```python
from build123d import *

# Parameters (mm, degrees)
SKETCH_1_W          = 20
SKETCH_1_H          = 10
EXTRUDE_1_DEPTH     = 3
SKETCH_2_W          = 20
SKETCH_2_H          = 3
EXTRUDE_2_DEPTH     = 18
SKETCH_3_W          = 16
SKETCH_3_H          = 12
CUT_EXTRUDE_1_DEPTH = 8
EXTRUDE_3_DEPTH     = 3
SKETCH_5_R          = 1.05
CUT_EXTRUDE_2_DEPTH = 10
FILLET_2_R          = 1
FILLET_3_R          = 1
FILLET_4_R          = 1
SKETCH_6_W          = 20
SKETCH_6_H          = 21
CUT_EXTRUDE_3_DEPTH = 10
SKETCH_7_W          = 24
SKETCH_7_H          = 24
EXTRUDE_4_DEPTH     = 3
SKETCH_8_W          = 24
SKETCH_8_H          = 3
EXTRUDE_5_DEPTH     = 7
SKETCH_9_W          = 20
SKETCH_9_H          = 18
CUT_EXTRUDE_4_DEPTH = 7
SKETCH_10_W         = 32
SKETCH_10_H         = 7
EXTRUDE_6_DEPTH     = 3
SKETCH_11_R         = 1.1
CUT_EXTRUDE_5_DEPTH = 4


with BuildPart() as part:
    # 草图1 → 凸台-拉伸1 (new body)
    with BuildSketch(Plane.XY):
        with Locations((10, 5)):
            Rectangle(SKETCH_1_W, SKETCH_1_H)
    extrude(amount=EXTRUDE_1_DEPTH)

    # 草图2 → 凸台-拉伸2 (add)
    with BuildSketch(Plane.XY.offset(3)):
        with Locations((10, 8.5)):
            Rectangle(SKETCH_2_W, SKETCH_2_H)
    extrude(amount=EXTRUDE_2_DEPTH)

    # 草图3 → 切除-拉伸1 (cut)
    with BuildSketch(Plane.XZ.offset(-7)):
        with Locations((10, 12)):
            Rectangle(SKETCH_3_W, SKETCH_3_H)
    extrude(amount=-CUT_EXTRUDE_1_DEPTH, mode=Mode.SUBTRACT)

    # 草图4 → 凸台-拉伸3 (add)
    with BuildSketch(Plane.XZ.offset(-7)):
        Polygon((0, 21), (-3.5, 21), (-3.5, 38), (23.5, 38), (23.5, 21), align=None)
    extrude(amount=-EXTRUDE_3_DEPTH)

    # 草图5 → 切除-拉伸2 (cut)
    with BuildSketch(Plane.XZ.offset(-7)):
        with Locations((-0.5, 23.5)):
            Circle(SKETCH_5_R)
        with Locations((20.5, 23.5)):
            Circle(SKETCH_5_R)
        with Locations((20.5, 35.5)):
            Circle(SKETCH_5_R)
        with Locations((-0.5, 35.5)):
            Circle(SKETCH_5_R)
    extrude(amount=-CUT_EXTRUDE_2_DEPTH, mode=Mode.SUBTRACT)

    # 圆角2
    fillet_2_edges = [part.edges().sort_by_distance(p)[0] for p in [
        (10, 0, 3),
    ]]
    fillet(fillet_2_edges, radius=FILLET_2_R)

    # 圆角3
    fillet_3_edges = [part.edges().sort_by_distance(p)[0] for p in [
        (0, 4, 3),
        (20, 4, 3),
        (20, 0, 1),
        (20, 0.292893219, 2.707106781),
        (0, 0, 1),
        (0, 0.292893219, 2.707106781),
    ]]
    fillet(fillet_3_edges, radius=FILLET_3_R)

    # 圆角4
    fillet_4_edges = [part.edges().sort_by_distance(p)[0] for p in [
        (2, 7, 12),
        (10, 7, 6),
        (18, 7, 12),
        (10, 7, 18),
    ]]
    fillet(fillet_4_edges, radius=FILLET_4_R)

    # 草图6 → 切除-拉伸3 (cut)
    with BuildSketch(Plane(origin=(0, 10, 0), x_dir=(1, 0, 0), z_dir=(0, 1, 0))):
        with Locations((10, -10.5)):
            Rectangle(SKETCH_6_W, SKETCH_6_H)
    extrude(amount=-CUT_EXTRUDE_3_DEPTH, mode=Mode.SUBTRACT)

    # 草图7 → 凸台-拉伸4 (add)
    with BuildSketch(Plane(origin=(0, 10, 0), x_dir=(1, 0, 0), z_dir=(0, 1, 0))):
        with Locations((10, -9)):
            Rectangle(SKETCH_7_W, SKETCH_7_H)
    extrude(amount=-EXTRUDE_4_DEPTH)

    # 草图8 → 凸台-拉伸5 (add)
    with BuildSketch(Plane.XZ.offset(-7)):
        with Locations((10, -1.5)):
            Rectangle(SKETCH_8_W, SKETCH_8_H)
    extrude(amount=EXTRUDE_5_DEPTH)

    # 草图9 → 切除-拉伸4 (cut)
    with BuildSketch(Plane(origin=(0, 10, 0), x_dir=(1, 0, 0), z_dir=(0, 1, 0))):
        with Locations((10, -11)):
            Rectangle(SKETCH_9_W, SKETCH_9_H)
    extrude(amount=-CUT_EXTRUDE_4_DEPTH, mode=Mode.SUBTRACT)

    # 草图10 → 凸台-拉伸6 (add)
    with BuildSketch(Plane(origin=(0, 10, 0), x_dir=(1, 0, 0), z_dir=(0, 1, 0))):
        with Locations((10, 6.5)):
            Rectangle(SKETCH_10_W, SKETCH_10_H)
    extrude(amount=-EXTRUDE_6_DEPTH)

    # 草图11 → 切除-拉伸5 (cut)
    with BuildSketch(Plane(origin=(0, 10, 0), x_dir=(1, 0, 0), z_dir=(0, 1, 0))):
        with Locations((-4.2, 7)):
            Circle(SKETCH_11_R)
        with Locations((24.2, 7)):
            Circle(SKETCH_11_R)
    extrude(amount=-CUT_EXTRUDE_5_DEPTH, mode=Mode.SUBTRACT)


solid = part.part
```
Here's how the part is built. I have some questions about the finished solid (model axes, mm). A direction names the side the tool comes from. Coordinates: 2 decimals unless noted, no trailing zeros. Order: outer loops, then holes, each group sorted by start corner. A loop starts at its lowest first (then second) coordinate and runs counter-clockwise, first axis right, second up.
1) Imagine slicing it at D-D on x = 24.2. List the corners of the cut face in (y, z) for me, and give its area (3 significant figures).
2) I need wall thicknesses on line 1 (X direction, y = 9.15, z = -7); line 2 (Z direction, x = 20.5, y = 8); line 3 (X direction, y = 9.5, z = 15). Which ranges of each line are inside material? Lowest first, please.
3) Will these pins go through, and if not, where does the flat tip stop? pin 1 (1.7 mm diameter, centred on x = -0.5, z = 35.5, fed in from -Y); pin 2 (1.5 mm diameter, centred on y = 6.5, z = 30, fed in from +X); pin 3 (3.5 mm diameter, centred on y = 9, z = 29, fed in from -X); pin 4 (1.5 mm diameter, centred on y = 9, z = 12, fed in from -X).
4) Imagine slicing it at A-A on z = 23.5. List the corners of the cut face in (x, y) for me, and give its area (3 significant figures).
5) Imagine slicing it at C-C on y = 9. List the corners of the cut face in (x, z) for me.
6) We'd pull the mould along Z, two halves only. Please class faces 1 (the face through (10, 4, 0)), 2 (the face through (10, 7, 28)), 3 (the face through (-1.33, 8.48, 34.86)): +Z half, -Z half, draft (parallel to the pull), parting line (faces both ways), or undercut.
7) Which directions (+Z, -Z, +X, -X, +Y, -Y) give clear straight access to the entire face, cutting with the end or side of a thin tool? Please do faces 4 (the face through (10, 4, -3)), 5 (the face through (10, 9, 20)), 6 (the face through (24, 9, -3)), 7 (the face through (-3.5, 8, 29)).
8) Imagine slicing it at B-B on x = 20.5. List the corners of the cut face in (y, z) for me.
Response values:
1. outline: (7, -10) - (10, -10) - (10, -8.1) - (7, -8.1) - close; (7, -5.9) - (10, -5.9) - (10, -3) - (7, -3) - close
1. area: 14.4 mm2
2. line 1: x = -6 to -5.3, -3.1 to 23.1, 25.3 to 26
2. line 2: z = -10 to 22.45, 24.55 to 34.45, 36.55 to 38
2. line 3: x = -2 to 0, 20 to 22
3. pin 1: passes through
3. pin 2: stops at x = 23.5
3. pin 3: stops at x = -3.5
3. pin 4: stops at x = -2
4. outline: (-3.5, 7) - (-1.55, 7) - (-1.55, 10) - (-3.5, 10) - close; (0.55, 7) - (19.45, 7) - (19.45, 10) - (0.55, 10) - close; (21.55, 7) - (23.5, 7) - (23.5, 10) - (21.55, 10) - close
4. area: 68.4 mm2
5. outline: (-6, -10) - (26, -10) - (26, -3) - (22, -3) - (22, 21) - (23.5, 21) - (23.5, 38) - (-3.5, 38) - (-3.5, 21) - (-2, 21) - (-2, -3) - (-6, -3) - close; hole circle Ø2.2 at (-4.2, -7); hole circle Ø2.1 at (-0.5, 23.5); hole circle Ø2.1 at (-0.5, 35.5); hole (0, 2) - (20, 2) - (20, 20) - (0, 20) - close; hole circle Ø2.1 at (20.5, 23.5); hole circle Ø2.1 at (20.5, 35.5); hole circle Ø2.2 at (24.2, -7)
6. face 1: +Z half
6. face 2: draft
6. face 3: undercut
7. face 4: -Z, +X, -X, -Y
7. face 5: +Y, -Y
7. face 6: +X, +Y, -Y
7. face 7: +Z, -X, +Y, -Y
8. outline: (0, -3) - (7, -3) - (7, -10) - (10, -10) - (10, 22.45) - (7, 22.45) - (7, 0) - (0, 0) - close; (7, 24.55) - (10, 24.55) - (10, 34.45) - (7, 34.45) - close; (7, 36.55) - (10, 36.55) - (10, 38) - (7, 38) - close
